Geometry check sheet. Reference: the model listing, model coordinates, mm. A direction names the side the tool comes from. Coordinates: 2 decimals unless noted, no trailing zeros. Order: outer loops, then holes, each group sorted by start corner. A loop starts at its lowest first (then second) coordinate and runs counter-clockwise, first axis right, second up. Notation, with made-up numbers: (-15.75, 0) -> (40.25, 0) arc R20 ccw to (40.25, 21) -> close; hole circle Ø1 at (2.5, 11). An arc over 180 degrees is marked (long way). Answer in a Markdown table with one row per item. Add a question column.
```python
from build123d import *

# Parameters (mm, degrees)
SALIENTE_EXTRUIR1_DEPTH = 40
CORTAR_EXTRUIR1_REACH   = 71.282
CROQUIS2_R              = 2.25
REDONDEO3_R             = 4
CROQUIS3_R              = 4.15
CORTAR_EXTRUIR3_DEPTH   = 25
CORTAR_EXTRUIR5_DEPTH   = 1
CROQUIS7_R              = 2.65
CORTAR_EXTRUIR6_DEPTH   = 70.28203236


with BuildPart() as part:
    # Croquis1 → Saliente-Extruir1 (new body)
    with BuildSketch(Plane(origin=(0, 0, 0), x_dir=(1, 0, 0), z_dir=(0, 1, 0))):
        Polygon((0, 0), (40, 0), (40, 20), (20, 20), (20, 40), (0, 40), align=None)
    extrude(amount=SALIENTE_EXTRUIR1_DEPTH)

    # Croquis2 → Cortar-Extruir1 (cut, up to next)
    with BuildSketch(Plane(origin=(0, 40, 0), x_dir=(1, 0, 0), z_dir=(0, 1, 0)), mode=Mode.PRIVATE) as cortar_extruir1_sk1:
        with Locations(Location((30, 10, 0), (0, 0, 270))):
            Circle(CROQUIS2_R)
    cortar_extruir1_tool1 = extrude(cortar_extruir1_sk1.sketch, amount=-CORTAR_EXTRUIR1_REACH, mode=Mode.PRIVATE) & part.part
    # Croquis2 → Cortar-Extruir1 (cut, up to next)
    with BuildSketch(Plane(origin=(0, 40, 0), x_dir=(1, 0, 0), z_dir=(0, 1, 0)), mode=Mode.PRIVATE) as cortar_extruir1_sk2:
        with Locations(Location((10, 10, 0), (0, 0, 270))):
            Circle(CROQUIS2_R)
    cortar_extruir1_tool2 = extrude(cortar_extruir1_sk2.sketch, amount=-CORTAR_EXTRUIR1_REACH, mode=Mode.PRIVATE) & part.part
    add(cortar_extruir1_tool1.solids().sort_by_distance((30, 40, -10))[0], mode=Mode.SUBTRACT)
    add(cortar_extruir1_tool2.solids().sort_by_distance((10, 40, -10))[0], mode=Mode.SUBTRACT)

    # Redondeo3
    redondeo3_edges = [part.edges().sort_by_distance(p)[0] for p in [
        (40, 40, -10),
        (0, 20, -40),
        (20, 20, -40),
        (20, 20, -20),
        (40, 20, -20),
        (40, 20, 0),
        (0, 20, 0),
        (30, 40, -20),
        (20, 40, -30),
        (10, 40, -40),
        (0, 40, -20),
        (20, 40, 0),
    ]]
    fillet(redondeo3_edges, radius=REDONDEO3_R)

    # Croquis3 → Cortar-Extruir3 (cut)
    with BuildSketch(Plane(origin=(0, 0, -40), x_dir=(-1, 0, 0), z_dir=(0, 0, -1))):
        with Locations((-10, 30)):
            Circle(CROQUIS3_R)
    extrude(amount=-CORTAR_EXTRUIR3_DEPTH, mode=Mode.SUBTRACT)

    # Croquis6 → Cortar-Extruir5 (cut)
    with BuildSketch(Plane(origin=(0, 40, 0), x_dir=(1, 0, 0), z_dir=(0, 1, 0))):
        with BuildLine():
            Line((18.692307692, 10.607697294), (18.153846154, 10.607697294))
            add(Edge.make_bspline(
                [(18.153846154, 10.607697294), (18.168433955, 10.668095838), (18.196951913, 10.786170051), (18.256433468, 10.954868213), (18.321232191, 11.114508535), (18.399042084, 11.262101804), (18.483914234, 11.400614209), (18.581153186, 11.526904137), (18.68627271, 11.644183506), (18.802544052, 11.748263342), (18.9244789, 11.842510878), (19.053795391, 11.922868119), (19.18789178, 11.991995238), (19.327697151, 12.048944207), (19.473627731, 12.091845105), (19.624364228, 12.122971057), (19.780301657, 12.143184396), (19.88615467, 12.145157132), (19.939903846, 12.146158832)],
                knots=[0, 0, 0, 0, 1.162005537, 2.271625781, 3.343758855, 4.383309926, 5.390229558, 6.379919256, 7.361854164, 8.333198761, 9.295911338, 10.242430842, 11.177959212, 12.116337295, 13.062827104, 14.020064771, 14.994644689, 16, 16, 16, 16], degree=3))
            add(Edge.make_bspline(
                [(19.939903846, 12.146158832), (20.018217118, 12.143794438), (20.173135423, 12.139117223), (20.400729218, 12.09640676), (20.620203765, 12.028820819), (20.829156761, 11.935437287), (21.023245502, 11.820259036), (21.195936108, 11.683176629), (21.344887841, 11.52683497), (21.469849631, 11.354150574), (21.567692487, 11.169598272), (21.639840556, 10.979655145), (21.683763437, 10.784771766), (21.689455821, 10.653187859), (21.692307692, 10.587264602)],
                knots=[0, 0, 0, 0, 1.083050992, 2.142477498, 3.193116406, 4.255571735, 5.30263384, 6.308962982, 7.297363603, 8.282367274, 9.249857812, 10.179914175, 11.08814088, 12, 12, 12, 12], degree=3))
            add(Edge.make_bspline(
                [(21.692307692, 10.587264602), (21.690312965, 10.523824382), (21.686409593, 10.399681717), (21.653266097, 10.218444865), (21.597489647, 10.047630693), (21.520227197, 9.88652013), (21.42021311, 9.73613469), (21.299059916, 9.59613602), (21.155912496, 9.465903177), (21.047434316, 9.391298367), (20.991586538, 9.352889602)],
                knots=[0, 0, 0, 0, 1.024540389, 2.004866551, 2.965041327, 3.920577974, 4.882998113, 5.874504559, 6.905732034, 8, 8, 8, 8], degree=3))
            add(Edge.make_bspline(
                [(20.991586538, 9.352889602), (21.055412403, 9.322069879), (21.181869902, 9.261007095), (21.354242239, 9.141254367), (21.510718596, 9.002986343), (21.597982115, 8.895084653), (21.641826923, 8.840870371)],
                knots=[0, 0, 0, 0, 1.015518401, 2.012035669, 3.001164323, 4, 4, 4, 4], degree=3))
            add(Edge.make_bspline(
                [(21.641826923, 8.840870371), (21.670697796, 8.801342797), (21.72796676, 8.72293494), (21.798656247, 8.596872495), (21.862786157, 8.469412799), (21.912757962, 8.337139532), (21.951456019, 8.201585794), (21.979117789, 8.06251883), (21.99630203, 7.919825077), (21.998762976, 7.823289396), (22, 7.774764602)],
                knots=[0, 0, 0, 0, 1.025084078, 2.033381695, 3.024893161, 4.013698104, 4.991890475, 5.976764909, 6.982997093, 8, 8, 8, 8], degree=3))
            add(Edge.make_bspline(
                [(22, 7.774764602), (21.996923691, 7.690747937), (21.99078555, 7.523109991), (21.935921423, 7.275439039), (21.850870153, 7.033338178), (21.730086835, 6.801781311), (21.582885391, 6.585129229), (21.407758549, 6.391284128), (21.206696135, 6.224657949), (20.98245788, 6.085440416), (20.739514231, 5.974152549), (20.479670359, 5.896911218), (20.206670266, 5.84660379), (20.019457756, 5.841209158), (19.924278846, 5.838466525)],
                knots=[0, 0, 0, 0, 0.955779014, 1.907060117, 2.875433937, 3.871313158, 4.872415639, 5.851225146, 6.836215519, 7.83643374, 8.849228613, 9.86973379, 10.916971861, 12, 12, 12, 12], degree=3))
            add(Edge.make_bspline(
                [(19.924278846, 5.838466525), (19.860131474, 5.83995489), (19.733910837, 5.842883498), (19.548350554, 5.862903957), (19.371227641, 5.89946968), (19.202302616, 5.948675346), (19.041425411, 6.01106119), (18.889086945, 6.088750387), (18.744349984, 6.180141533), (18.608580354, 6.286313398), (18.481794238, 6.405081409), (18.367360996, 6.538553997), (18.26337278, 6.684263833), (18.172613971, 6.843903357), (18.090950623, 7.015409513), (18.023783269, 7.200978367), (17.964665151, 7.398950976), (17.937179213, 7.536912817), (17.923076923, 7.607697294)],
                knots=[0, 0, 0, 0, 1.048658725, 2.063410685, 3.046034179, 4.001477787, 4.936774919, 5.862367409, 6.792675028, 7.730719943, 8.675894397, 9.627829632, 10.600096036, 11.597688215, 12.626045268, 13.701542398, 14.82072376, 16, 16, 16, 16], degree=3))
            Line((17.923076923, 7.607697294), (18.461538462, 7.607697294))
            add(Edge.make_bspline(
                [(18.461538462, 7.607697294), (18.475566961, 7.561498986), (18.502853611, 7.471639263), (18.549300979, 7.342313024), (18.602218017, 7.223756362), (18.658985832, 7.115099581), (18.718606025, 7.015272606), (18.785317326, 6.926915116), (18.854178717, 6.846146198), (18.90608618, 6.800641149), (18.931490385, 6.778370371)],
                knots=[0, 0, 0, 0, 1.198163088, 2.33053128, 3.407730985, 4.417276592, 5.372219308, 6.28897303, 7.162600585, 8, 8, 8, 8], degree=3))
            add(Edge.make_bspline(
                [(18.931490385, 6.778370371), (18.965084516, 6.75247037), (19.032169081, 6.700750315), (19.141486048, 6.634747524), (19.256454424, 6.577557195), (19.379565295, 6.533870859), (19.508162044, 6.496880583), (19.644323241, 6.472673979), (19.786847614, 6.456065685), (19.88416378, 6.454600089), (19.933894231, 6.45385114)],
                knots=[0, 0, 0, 0, 0.946170439, 1.889420265, 2.845303464, 3.807233317, 4.801018734, 5.828864929, 6.890507805, 8, 8, 8, 8], degree=3))
            add(Edge.make_bspline(
                [(19.933894231, 6.45385114), (19.990043092, 6.454906978), (20.099837344, 6.456971577), (20.260045675, 6.475958503), (20.412458442, 6.50361064), (20.555383457, 6.546318611), (20.690692899, 6.599085785), (20.816490012, 6.665340194), (20.934426194, 6.743074003), (21.042990889, 6.831426846), (21.140611759, 6.928149409), (21.226565211, 7.029314674), (21.299636059, 7.134496096), (21.358579336, 7.244275732), (21.405123136, 7.358198981), (21.436808623, 7.476585546), (21.458839792, 7.598466574), (21.460633984, 7.681316235), (21.461538462, 7.723081909)],
                knots=[0, 0, 0, 0, 1.217147791, 2.380027433, 3.494444702, 4.572153297, 5.609568379, 6.639424714, 7.649109417, 8.668170816, 9.669597737, 10.625200337, 11.543417969, 12.441394052, 13.322311151, 14.205496177, 15.095365482, 16, 16, 16, 16], degree=3))
            add(Edge.make_bspline(
                [(21.461538462, 7.723081909), (21.458915087, 7.778987062), (21.453681393, 7.89051919), (21.413723828, 8.05460646), (21.348000061, 8.212703739), (21.255990042, 8.362113665), (21.143985935, 8.500586639), (21.013074666, 8.624137752), (20.862169132, 8.726086479), (20.723277928, 8.796524176), (20.600251945, 8.844587733), (20.494968429, 8.876601958), (20.377099966, 8.903711082), (20.24807194, 8.928932119), (20.10691214, 8.950397287), (19.953774246, 8.968297543), (19.788627227, 8.98262047), (19.674299514, 8.989016633), (19.615384615, 8.992312679)],
                knots=[0, 0, 0, 0, 1.07054697, 2.135767047, 3.216561865, 4.33974944, 5.486079747, 6.621378074, 7.775625952, 8.963672916, 9.598146892, 10.304877434, 11.070270905, 11.915000392, 12.823868403, 13.805723172, 14.86925407, 16, 16, 16, 16], degree=3))
            Line((19.615384615, 8.992312679), (19.615384615, 9.607697294))
            add(Edge.make_bspline(
                [(19.615384615, 9.607697294), (19.689615185, 9.608956958), (19.835014636, 9.611424329), (20.047404873, 9.641266632), (20.25050198, 9.682547709), (20.439804966, 9.745779467), (20.612345617, 9.819219976), (20.762036364, 9.904680907), (20.886780045, 9.99967762), (20.985970453, 10.105676379), (21.060591988, 10.219359317), (21.115152212, 10.337845016), (21.147381343, 10.462171978), (21.151683629, 10.54701998), (21.153846154, 10.589668448)],
                knots=[0, 0, 0, 0, 1.321986639, 2.589447074, 3.816329219, 5.01088745, 6.139805852, 7.153945165, 8.075214402, 8.924034688, 9.728124013, 10.488707548, 11.240355623, 12, 12, 12, 12], degree=3))
            add(Edge.make_bspline(
                [(21.153846154, 10.589668448), (21.153135735, 10.621001725), (21.151722391, 10.683337795), (21.133898486, 10.774409341), (21.107114416, 10.862696677), (21.070292022, 10.947824351), (21.021005968, 11.029201964), (20.962024276, 11.107523305), (20.891793247, 11.182341212), (20.811315338, 11.252078902), (20.724895101, 11.318540452), (20.630181201, 11.37496383), (20.530029416, 11.423212507), (20.424328865, 11.463000225), (20.312736527, 11.492930434), (20.195776714, 11.514420447), (20.073226399, 11.527856427), (19.989617716, 11.529790854), (19.947115385, 11.530774217)],
                knots=[0, 0, 0, 0, 0.884392785, 1.759457502, 2.611959086, 3.489218968, 4.37281399, 5.2945488, 6.255912374, 7.266815255, 8.301784654, 9.332968512, 10.37626691, 11.440494194, 12.520033166, 13.637162961, 14.798855837, 16, 16, 16, 16], degree=3))
            add(Edge.make_bspline(
                [(19.947115385, 11.530774217), (19.878798239, 11.528389025), (19.745358966, 11.52373019), (19.552990537, 11.482925024), (19.374157393, 11.417819738), (19.237462536, 11.340105991), (19.13652098, 11.263390961), (19.064389086, 11.196392585), (18.993553925, 11.121936316), (18.928675622, 11.035436244), (18.863063091, 10.942750318), (18.803329557, 10.839166864), (18.74528437, 10.727387902), (18.71030857, 10.648366814), (18.692307692, 10.607697294)],
                knots=[0, 0, 0, 0, 1.472543308, 2.876219568, 4.221790263, 5.565193594, 6.249813518, 6.953379497, 7.687249741, 8.463570142, 9.283606569, 10.136032583, 11.040678096, 12, 12, 12, 12], degree=3))
        make_face()
    extrude(amount=-CORTAR_EXTRUIR5_DEPTH, mode=Mode.SUBTRACT)

    # Croquis7 → Cortar-Extruir6 (cut, through all)
    with BuildSketch(Plane.ZY):
        with Locations((-26, 20)):
            Circle(CROQUIS7_R)
    extrude(amount=-CORTAR_EXTRUIR6_DEPTH, mode=Mode.SUBTRACT)


solid = part.part
```
(1) Go/stop test with flat-tipped pins: P1, Ø9.5, axis at x = 28.5, y = 9.5, coming from the -Z side; P2, Ø8.5, axis at y = 20, z = -26, coming from the +X side; P3, Ø9.5, axis at y = 15, z = -31.5, coming from the +X side; P4, Ø2.5, axis at x = 10, z = -10, coming from the -Y side. Record where each tip stops, or that it passes through.
(2) Cross-section at D-D (y = 35). Enter the section's corners in (x, z).
(3) Scan lines: line 1 along X through (y, z) = (31.5, -10); line 2 along X through (y, z) = (32, -12); line 3 along Y through (x, z) = (11, -26). Record each from-to range of solid material in increasing order.
(4) Access from +Z, -Z, +X, -X, +Y, -Y to the whole of each face (thin tool, end or side, straight path). Record for faces 5 (the face through (29.916, 38.859, -18.797)), 6 (the face through (30, 18, -20)), 7 (the face through (13.059, 32.805, -27.675)), 8 (the face through (40, 18, -10)).
(5) Cross-section at B-B (x = 30). Enter the section's corners in (y, z).
(6) Cross-section at A-A (y = 20). Enter the section's corners in (x, z), plus the area to 3 significant figures.
(7) Mould release check, pull along Y, two halves, no side actions. Record for faces 1 (the face through (0, 18, -20)), 2 (the face through (10, 30, -15)), 3 (the face through (9.886, 20.117, -28.647)), 4 (the face through (38.859, 38.797, -10.084)): +Y half, -Y half, draft (parallel to the pull), parting line (faces both ways), or undercut.
(8) Cross-section at C-C (z = -25.5). Enter the section's corners in (x, y).
Checks:
| question | item | result |
|---|---|---|
| 1 | P1 | z = -20.01 |
| 1 | P2 | x = 20.69 |
| 1 | P3 | x = 20 |
| 1 | P4 | through |
| 2 | outline | (0, -36) arc R4 ccw to (4, -40) -> (16, -40) arc R4 ccw to (20, -36) -> (20, -24) arc R4 cw to (24, -20) -> (36, -20) arc R4 ccw to (40, -16) -> (40, -4) arc R4 ccw to (36, 0) -> (4, 0) arc R4 ccw to (0, -4) -> close; hole circle Ø4.5 at (10, -10); hole circle Ø4.5 at (30, -10) |
| 3 | line 1 | 0 to 7.75, 12.25 to 27.75, 32.25 to 40 |
| 3 | line 2 | 0 to 8.97, 11.03 to 28.97, 31.03 to 40 |
| 3 | line 3 | 0 to 17.35, 22.65 to 25.97, 34.03 to 40 |
| 4 | face 5 | -Z, +X, +Y |
| 4 | face 6 | -Z, +X, +Y, -Y |
| 4 | face 7 | -Z |
| 4 | face 8 | +Z, -Z, +X, +Y, -Y |
| 5 | outline | (0, -20) -> (36, -20) arc R4 ccw to (40, -16) -> (40, -12.25) -> (0, -12.25) -> close; (0, -7.75) -> (40, -7.75) -> (40, -4) arc R4 ccw to (36, 0) -> (0, 0) -> close |
| 6 | outline | (0, -36) arc R4 ccw to (4, -40) -> (16, -40) arc R4 ccw to (20, -36) -> (20, -28.65) -> (0, -28.65) -> close; (0, -23.35) -> (20.05, -23.35) arc R4 cw to (24, -20) -> (36, -20) arc R4 ccw to (40, -16) -> (40, -4) arc R4 ccw to (36, 0) -> (4, 0) arc R4 ccw to (0, -4) -> close; hole circle Ø4.5 at (10, -10); hole circle Ø4.5 at (30, -10) |
| 6 | area | 1,050 mm² |
| 7 | face 1 | draft |
| 7 | face 2 | undercut |
| 7 | face 3 | undercut |
| 7 | face 4 | +Y half |
| 8 | outline | (0, 0) -> (20, 0) -> (20, 17.4) -> (0, 17.4) -> close; (0, 22.6) -> (20, 22.6) -> (20, 36) arc R4 ccw to (16, 40) -> (4, 40) arc R4 ccw to (0, 36) -> close; hole circle Ø8.3 at (10, 30) |
